Can you work these out from the model? Positions are in its coordinate system, mm. Face numbers are marked on the shaded views. Give positions to 0.01 mm unless a question says otherwise; leave off trailing zeros. Loops run counter-clockwise (first coordinate to the right, second up) from the corner with the lowest first, then second, coordinate; pieces in that order, holes last. Notation, with made-up numbers: M -24.75,69.5 L 13.25,69.5 A28 cw 13.25,98.5 Z; hole C 78,-19.5 d5. An arc over 180 degrees is marked long. Answer as a JSON object with one key per item and string values.
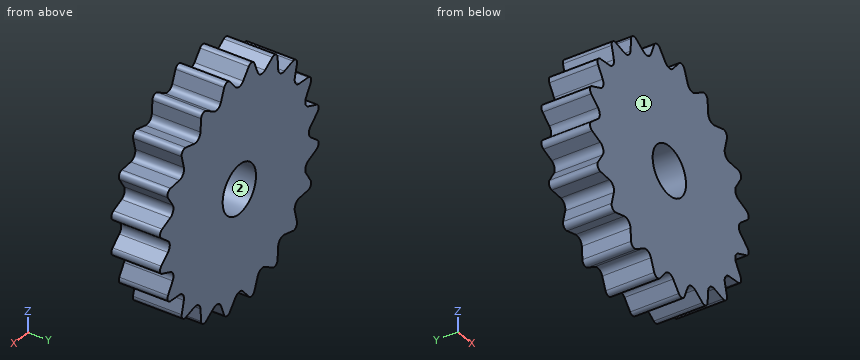
```python
from build123d import *

# Parameters (mm, degrees)
F0_R     = 6.35
F1_DEPTH = 12.7
F2_R     = 1.905
F3_R     = 1.27


with BuildPart() as f1:
    # F0 (on Front) → F1 (new body)
    with BuildSketch(Plane.XZ):
        Polygon((22.45064, 22.45064), (14.929745, 20.549032), (14.414198, 28.289457), (7.849032, 24.156836), (4.966794, 31.359105), (0, 25.4), (-4.966794, 31.359105), (-7.849032, 24.156836), (-14.414198, 28.289457), (-14.929745, 20.549032), (-22.45064, 22.45064), (-20.549032, 14.929745), (-28.289457, 14.414198), (-24.156836, 7.849032), (-31.359105, 4.966794), (-25.4, 0), (-31.359105, -4.966794), (-24.156836, -7.849032), (-28.289457, -14.414198), (-20.549032, -14.929745), (-22.45064, -22.45064), (-14.929745, -20.549032), (-14.414198, -28.289457), (-7.849032, -24.156836), (-4.966794, -31.359105), (0, -25.4), (4.966794, -31.359105), (7.849032, -24.156836), (14.414198, -28.289457), (14.929745, -20.549032), (22.45064, -22.45064), (20.549032, -14.929745), (28.289457, -14.414198), (24.156836, -7.849032), (31.359105, -4.966794), (25.4, 0), (31.359105, 4.966794), (24.156836, 7.849032), (28.289457, 14.414198), (20.549032, 14.929745), align=None)
        Circle(F0_R, mode=Mode.SUBTRACT)
    extrude(amount=F1_DEPTH)

    # F2
    f2_edges = [f1.edges().sort_by_distance(p)[0] for p in [
        (-20.549032, -6.35, 14.929745),
        (-14.929745, -6.35, 20.549032),
        (-24.156836, -6.35, 7.849032),
        (-25.4, -6.35, 0),
        (-24.156836, -6.35, -7.849032),
        (-20.549032, -6.35, -14.929745),
        (-14.929745, -6.35, -20.549032),
        (-7.849032, -6.35, -24.156836),
        (0, -6.35, -25.4),
        (7.849032, -6.35, -24.156836),
        (14.929745, -6.35, -20.549032),
        (20.549032, -6.35, -14.929745),
        (24.156836, -6.35, -7.849032),
        (25.4, -6.35, 0),
        (24.156836, -6.35, 7.849032),
        (20.549032, -6.35, 14.929745),
        (14.929745, -6.35, 20.549032),
        (7.849032, -6.35, 24.156836),
        (0, -6.35, 25.4),
        (-7.849032, -6.35, 24.156836),
    ]]
    fillet(f2_edges, radius=F2_R)

    # F3
    f3_edges = [f1.edges().sort_by_distance(p)[0] for p in [
        (28.289457, -6.35, -14.414198),
        (22.45064, -6.35, -22.45064),
        (14.414198, -6.35, -28.289457),
        (4.966794, -6.35, -31.359105),
        (-14.414198, -6.35, -28.289457),
        (-4.966794, -6.35, -31.359105),
        (-22.45064, -6.35, -22.45064),
        (-28.289457, -6.35, -14.414198),
        (-31.359105, -6.35, -4.966794),
        (-31.359105, -6.35, 4.966794),
        (-14.414198, -6.35, 28.289457),
        (-4.966794, -6.35, 31.359105),
        (-28.289457, -6.35, 14.414198),
        (-22.45064, -6.35, 22.45064),
        (4.966794, -6.35, 31.359105),
        (14.414198, -6.35, 28.289457),
        (22.45064, -6.35, 22.45064),
        (28.289457, -6.35, 14.414198),
        (31.359105, -6.35, 4.966794),
        (31.359105, -6.35, -4.966794),
    ]]
    fillet(f3_edges, radius=F3_R)


solid = f1.part
```
1) If we mould it in two halves opening along X, with no side actions, what happens to the marked faces 1 and 2? For each: +X half, -X half, draft (parallel to the pull), parting line (faces both ways), or undercut.
Answer list:
{"face 1": "draft", "face 2": "undercut"}
2) Suppose I cut it at A-A, the plane x = 0. Write out the boundary of the cut face in (y, z), and give its area (3 significant figures).
Answer list:
{"outline": "M -12.7,-26.47 L 0,-26.47 L 0,-6.35 L -12.7,-6.35 Z; M -12.7,6.35 L 0,6.35 L 0,26.47 L -12.7,26.47 Z", "area": "511 mm^2"}
3) Suppose I cut it at B-B, the plane z = 0. Write out the boundary of the cut face in (x, y), and give its area (3 significant figures).
Answer list:
{"outline": "M -26.47,-12.7 L -6.35,-12.7 L -6.35,0 L -26.47,0 Z; M 6.35,-12.7 L 26.47,-12.7 L 26.47,0 L 6.35,0 Z", "area": "511 mm^2"}
4) Please list where these lines run through material, in increasing order: line 1 along Z through (x, y) = (27, -1); line 2 along Z through (x, y) = (0, -3.5); line 3 along X through (y, z) = (-3, 23). Write a range as from..to.
Answer list:
{"line 1": "-14.16..-12.37, -6.71..-1.32, 1.32..6.71, 12.37..14.16", "line 2": "-26.47..-6.35, 6.35..26.47", "line 3": "-14.77..14.77"}
5) Suppose I cut it at C-C, the plane x = 16. Write out the boundary of the cut face in (y, z).
Answer list:
{"outline": "M -12.7,-21.18 L 0,-21.18 L 0,21.18 L -12.7,21.18 Z"}
6) Will these pins go through, and if not, where does the flat tip stop? pin 1 Ø2 at (y, z) = (-5.5, -10) entering from +X; pin 2 Ø2 at (y, z) = (-4, 23.5) entering from -X; pin 3 Ø2 at (x, y) = (-21, -3) entering from +Z.
Answer list:
{"pin 1": "x = 26.14", "pin 2": "x = -14.83", "pin 3": "z = 21.97"}
